from build123d import *

# Parameters (mm, degrees)
SKETCH1_R           = 3.5
BOSS_EXTRUDE1_DEPTH = 5
SKETCH2_R           = 20
BOSS_EXTRUDE2_DEPTH = 30
FILLET1_R           = 10
SKETCH3_R           = 10
BOSS_EXTRUDE3_DEPTH = 20
FILLET2_R           = 5
FILLET3_R           = 10


with BuildPart() as part:
    # Sketch1 → Boss-Extrude1 (new body)
    with BuildSketch(Plane(origin=(0, 0, 0), x_dir=(1, 0, 0), z_dir=(0, 1, 0))):
        with BuildLine():
            Line((-30, 40), (30, 40))
            ThreePointArc((30, 40), (37.071067812, 37.071067812), (40, 30))
            Line((40, 30), (40, -30))
            ThreePointArc((40, -30), (37.071067812, -37.071067812), (30, -40))
            Line((30, -40), (-30, -40))
            ThreePointArc((-30, -40), (-37.071067812, -37.071067812), (-40, -30))
            Line((-40, -30), (-40, 30))
            ThreePointArc((-40, 30), (-37.071067812, 37.071067812), (-30, 40))
        make_face()
        with Locations(Location((-28.284271247, 28.284271247, 0), (0, 0, 270))):
            Circle(SKETCH1_R, mode=Mode.SUBTRACT)
        with Locations(Location((28.284271247, 28.284271247, 0), (0, 0, 270))):
            Circle(SKETCH1_R, mode=Mode.SUBTRACT)
        with Locations(Location((28.284271247, -28.284271247, 0), (0, 0, 270))):
            Circle(SKETCH1_R, mode=Mode.SUBTRACT)
        with Locations(Location((-28.284271247, -28.284271247, 0), (0, 0, 270))):
            Circle(SKETCH1_R, mode=Mode.SUBTRACT)
    extrude(amount=BOSS_EXTRUDE1_DEPTH)

    # Sketch2 → Boss-Extrude2 (add)
    with BuildSketch(Plane(origin=(0, 5, 0), x_dir=(1, 0, 0), z_dir=(0, 1, 0))):
        with Locations(Location((0, 0, 0), (0, 0, 270))):
            Circle(SKETCH2_R)
    extrude(amount=BOSS_EXTRUDE2_DEPTH)

    # Fillet1
    fillet1_edges = [part.edges().sort_by_distance(p)[0] for p in [
        (0, 5, -20),
        (0, 35, -20),
    ]]
    fillet(fillet1_edges, radius=FILLET1_R)

    # Sketch3 → Boss-Extrude3 (add)
    with BuildSketch(Plane(origin=(0, 35, 0), x_dir=(1, 0, 0), z_dir=(0, 1, 0))):
        with Locations(Location((0, 0, 0), (0, 0, 270))):
            Circle(SKETCH3_R)
    extrude(amount=BOSS_EXTRUDE3_DEPTH)

    # Fillet2
    fillet2_edges = [part.edges().sort_by_distance(p)[0] for p in [
        (0, 35, -10),
    ]]
    fillet(fillet2_edges, radius=FILLET2_R)

    # Sketch4 → Revolve1 (revolve)
    with BuildSketch(Plane.XY):
        with BuildLine():
            Line((0, 50.392135624), (0, 87.892135624))
            ThreePointArc((0, 87.892135624), (18.75, 69.142135624), (0, 50.392135624))
        make_face()
    revolve(axis=Axis((0, 55, 0), (0, 1, 0)))

    # Fillet3
    fillet3_edges = [part.edges().sort_by_distance(p)[0] for p in [
        (-7.071067812, 53.281413698, -7.071067812),
    ]]
    fillet(fillet3_edges, radius=FILLET3_R)


solid = part.part
Can you work these out from the model? Positions are in its coordinate system, mm. A direction names the side the tool comes from. Round coordinates to 2 decimals unless told otherwise and drop trailing zeros. Loops run counter-clockwise (first coordinate to the right, second up) from the corner with the lowest first, then second, coordinate; pieces in that order, holes last. Notation, with made-up numbers: (45.5, 13.25) - (98.5, 13.25) arc R18 ccw to (98.5, 17.25) - close; hole circle Ø3 at (41.5, 24). An arc over 180 degrees is marked (long way). Answer in a Markdown table with one row per item. Add a question column.
Q1. I need wall thicknesses on L1, parallel to Y at x = 27, z = 34.5; L2, parallel to X at y = 13.5, z = 2; L3, parallel to Z at x = -9, y = 33.5. Which ranges of each line are inside material? Lowest first, please.
Q2. I want a section at A-A on y = 41.5. List the corners of the cut face in (x, z) for me.
Q3. I want a section at C-C on y = 57.5. List the corners of the cut face in (x, z) for me, and give its area (3 significant figures).
Q4. For pin 1 Ø5 at (y, z) = (31, 12) entering from -X; pin 2 Ø2 at (x, y) = (-2.5, 34.5) entering from -Z; pin 3 Ø8 at (x, y) = (13, 63) entering from -Z; pin 4 Ø5.5 at (x, z) = (28.28, 28.28) entering from -Y, each with a flat end and sliding along its axis, tell me the tip position at first contact or that it passes through.
Q5. Which directions (+Z, -Z, +X, -X, +Y, -Y) give clear straight access to the entire face, cutting with the end or side of a thin tool? Please do faces 1 (the flat face through (-40, 2, 0)), 2 (the cylindrical face through (-9.76, 43.75, -2.17)), 3 (the flat face through (18, 5, -27)).
Q6. We'd pull the mould along Z, two halves only. Please class faces 4 (the cylindrical face through (-19.524, 19.93, -4.336)), 5 (the flat face through (1, 0, -1)), 6 (the cylindrical face through (25.18, 2.46, 29.9)), 7 (the cylindrical face through (-36.99, 2.46, 37.15)): pulls with the +Z half, pulls with the -Z half, needs draft (parallel to the pull), parting line crosses it, or undercut.
Q7. I want a section at B-B on z = -34. List the corners of the cut face in (x, y) for me, and give its area (3 significant figures).
A:
| question | item | result |
|---|---|---|
| 1 | L1 | 0 to 5 |
| 1 | L2 | -20.01 to 20.01 |
| 1 | L3 | -12.33 to 12.33 |
| 2 | outline | circle Ø20 at (0, 0) |
| 3 | outline | circle Ø29.4 at (0, 0) |
| 3 | area | 679 mm^2 |
| 4 | pin 1 | x = -16.08 |
| 4 | pin 2 | z = -15.07 |
| 4 | pin 3 | z = -15.62 |
| 4 | pin 4 | through |
| 5 | face 1 | +Z, -Z, -X, +Y, -Y |
| 5 | face 2 | none |
| 5 | face 3 | +Y |
| 6 | face 4 | parting line crosses it |
| 6 | face 5 | needs draft |
| 6 | face 6 | undercut |
| 6 | face 7 | pulls with the +Z half |
| 7 | outline | (-39.17, 0) - (39.17, 0) - (39.17, 5) - (-39.17, 5) - close |
| 7 | area | 392 mm^2 |
